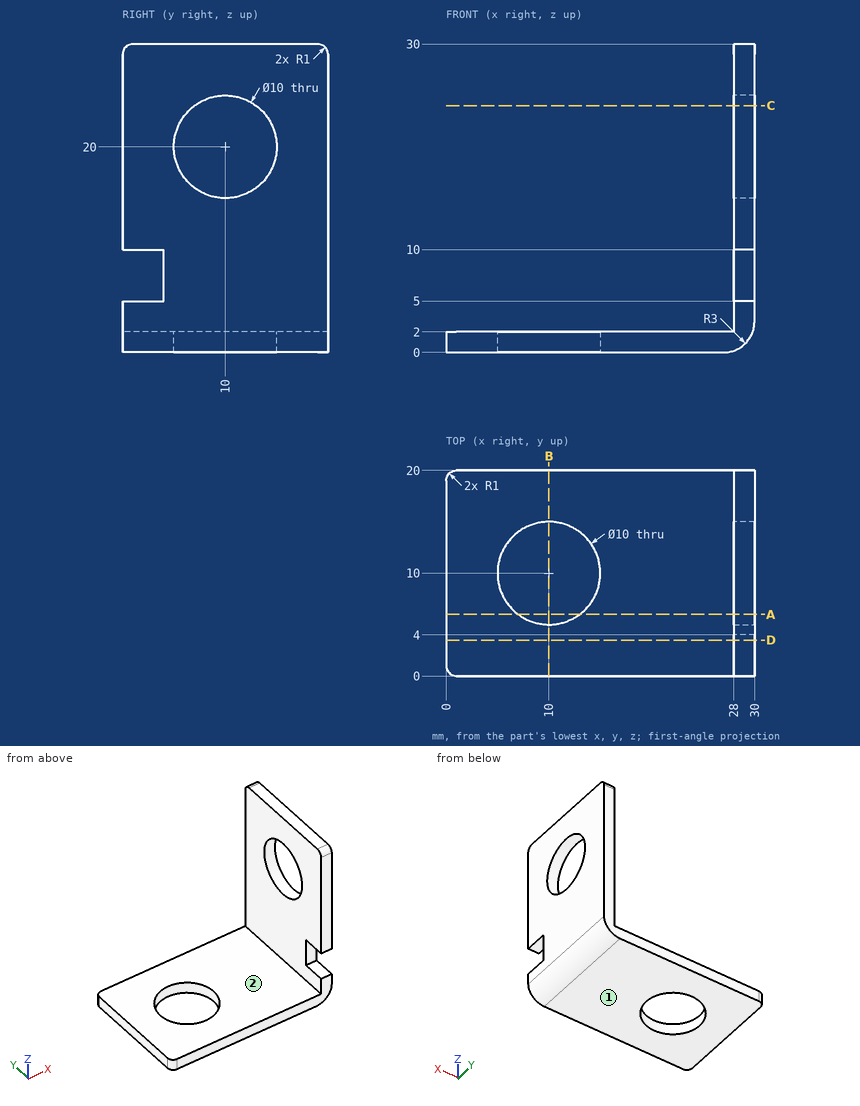
Geometry check sheet. Reference: drawing and pictorial views, mm from the part's lowest x, y, z. A direction names the side the tool comes from. Coordinates: 2 decimals unless noted, no trailing zeros. Write each loop counter-clockwise with the first axis right and the second up, starting at its lowest first coordinate (ties: lowest second). Pieces come first, ordered by that corner, then holes. Notation, with made-up numbers: (-34, 55.5) - (15, 55.5) arc R18 cw to (15, 67.5) - close; hole circle Ø9 at (60, 62.25). An arc over 180 degrees is marked (long way). Write item = value, one per line.
Q1. Cross-section at C-C (z = 24). Enter the section's corners in (x, y).
Answer:
outline = (28, 0) - (30, 0) - (30, 7) - (28, 7) - close; (28, 13) - (30, 13) - (30, 20) - (28, 20) - close
Q2. Cross-section at A-A (y = 6). Enter the section's corners in (x, z).
Answer:
outline = (0, 0) - (7, 0) - (7, 2) - (0, 2) - close; (13, 0) - (27, 0) arc R3 ccw to (30, 3) - (30, 17) - (28, 17) - (28, 2) - (13, 2) - close; (28, 23) - (30, 23) - (30, 30) - (28, 30) - close
Q3. Cross-section at B-B (x = 10). Enter the section's corners in (y, z), plus the area to 3 significant figures.
Answer:
outline = (0, 0) - (5, 0) - (5, 2) - (0, 2) - close; (15, 0) - (20, 0) - (20, 2) - (15, 2) - close
area = 20.0 mm²
Q4. Material ranges on L1, parallel to Y at x = 10, z = 1.65; L2, parallel to Z at x = 19.25, y = 15; L3, parallel to X at y = 14.75, z = 8.5, recorded low to high. Write a range as from..to.
Answer:
L1 = 0..5, 15..20
L2 = 0..2
L3 = 28..30
Q5. Cross-section at D-D (y = 3.5). Enter the section's corners in (x, z).
Answer:
outline = (0, 0) - (27, 0) arc R3 ccw to (30, 3) - (30, 5) - (28, 5) - (28, 2) - (0, 2) - close; (28, 10) - (30, 10) - (30, 30) - (28, 30) - close
Q6. Go/stop test with flat-tipped pins: pin 1 Ø1.6 at (x, z) = (29, 8) entering from -Y; pin 2 Ø6 at (x, y) = (19.5, 12.5) entering from +Z; pin 3 Ø2 at (x, y) = (28.5, 2.5) entering from -Z. Record where each tip stops, or that it passes through.
Answer:
pin_1 = 4
pin_2 = 2
pin_3 = 0.04
Q7. Access from +Z, -Z, +X, -X, +Y, -Y to the whole of each face (thin tool, end or side, straight path). Record for the marked faces 1 and 2.
Answer:
face_1 = -Z, +X, -X, +Y, -Y
face_2 = +Z, -X, +Y, -Y
